from build123d import *

# Parameters (mm, degrees)
SKETCH1_W                = 30
SKETCH1_H                = 22
BOSS_EXTRUDE1_DEPTH      = 11
SKETCH2_W                = 26.5
SKETCH2_H                = 18.5
CUT_EXTRUDE1_DEPTH       = 8
SKETCH3_R                = 1.2
BOSS_EXTRUDE2_DEPTH      = 3
CUT_EXTRUDE2_DEPTH       = 2
SKETCH5_W                = 7.639048366
SKETCH5_H                = 4
CUT_EXTRUDE3_DEPTH       = 34.793490497
CUT_EXTRUDE4_REACH       = 30.81
SKETCH6_W                = 26.5
SKETCH6_H                = 2
SKETCH8_W                = 24.775890618
SKETCH8_H                = 8.79217469
CUT_EXTRUDE5_DEPTH       = 2
FILLET1_R                = 3
SKETCH10_R               = 7
SKETCH10_R_2             = 5
BOSS_EXTRUDE4_DEPTH      = 8
BOSS_EXTRUDE8_REACH      = 36.471
BOSS_EXTRUDE8_END_RADIUS = 7
SKETCH15_W               = 8
SKETCH15_H               = 10
SKETCH16_W               = 7.639048366
SKETCH16_H               = 4
CUT_EXTRUDE7_DEPTH       = 46.861094623
CUT_EXTRUDE8_REACH       = 47.861


with BuildPart() as part:
    # Sketch1 → Boss-Extrude1 (new body)
    with BuildSketch(Plane(origin=(0, 0, 0), x_dir=(1, 0, 0), z_dir=(0, 1, 0))):
        Rectangle(SKETCH1_W, SKETCH1_H)
    extrude(amount=BOSS_EXTRUDE1_DEPTH)

    # Sketch2 → Cut-Extrude1 (cut)
    with BuildSketch(Plane(origin=(0, 11, 0), x_dir=(1, 0, 0), z_dir=(0, 1, 0))):
        Rectangle(SKETCH2_W, SKETCH2_H)
    extrude(amount=-CUT_EXTRUDE1_DEPTH, mode=Mode.SUBTRACT)

    # Sketch3 → Boss-Extrude2 (add)
    with BuildSketch(Plane(origin=(0, 3, 0), x_dir=(1, 0, 0), z_dir=(0, 1, 0))):
        with Locations(Location((-10.25, -6.3, 0), (0, 0, 90))):
            Circle(SKETCH3_R)
        with Locations(Location((10.25, -6.3, 0), (0, 0, 90))):
            Circle(SKETCH3_R)
        with Locations(Location((10.25, 6.3, 0), (0, 0, 90))):
            Circle(SKETCH3_R)
        with Locations(Location((-10.25, 6.3, 0), (0, 0, 90))):
            Circle(SKETCH3_R)
    extrude(amount=BOSS_EXTRUDE2_DEPTH)

    # Sketch4 → Cut-Extrude2 (cut)
    with BuildSketch(Plane(origin=(0, 3, 0), x_dir=(1, 0, 0), z_dir=(0, 1, 0))):
        Polygon((8.552738998, 7.070702511), (8.552738998, 5.36723461), (-8.55, 5.429297489), (-8.55, 7.070702511), align=None)
    cut_extrude2 = extrude(amount=-CUT_EXTRUDE2_DEPTH, mode=Mode.SUBTRACT)

    # Mirror1: Cut-Extrude2 across plane
    add(cut_extrude2.mirror(Plane.XY), mode=Mode.SUBTRACT)

    # Sketch5 → Cut-Extrude3 (cut, through all)
    with BuildSketch(Plane.ZY.offset(15)):
        with Locations((0, 6.5)):
            Rectangle(SKETCH5_W, SKETCH5_H)
    extrude(amount=-CUT_EXTRUDE3_DEPTH, mode=Mode.SUBTRACT)

    # Sketch6 → Cut-Extrude4 (cut, up to next)
    with BuildSketch(Plane.XY.offset(11), mode=Mode.PRIVATE) as cut_extrude4_sk1:
        with Locations((0, 9)):
            Rectangle(SKETCH6_W, SKETCH6_H)
    cut_extrude4_tool1 = extrude(cut_extrude4_sk1.sketch, amount=-CUT_EXTRUDE4_REACH, mode=Mode.PRIVATE) & part.part
    add(cut_extrude4_tool1.solids().sort_by_distance((0, 9, 11))[0], mode=Mode.SUBTRACT)

    # Sketch8 → Cut-Extrude5 (cut)
    with BuildSketch(Plane(origin=(0, 3, 0), x_dir=(1, 0, 0), z_dir=(0, 1, 0))):
        Rectangle(SKETCH8_W, SKETCH8_H)
    extrude(amount=-CUT_EXTRUDE5_DEPTH, mode=Mode.SUBTRACT)

    # Fillet1
    # the kernel refuses this fillet: 3 mm, written as the material it takes off along each edge
    with BuildSketch(Plane(origin=(-15, -7.5, 11), x_dir=(1, 0, 0), z_dir=(0, 1, 0)), Plane(origin=(-15, -7.5, -11), x_dir=(0, 0, 1), z_dir=(0, 1, 0))) as fillet1_piece_1:
        with BuildLine():
            CenterArc((FILLET1_R, FILLET1_R), FILLET1_R, 180, 90)
            Line((0, FILLET1_R), (0, 0))
            Line((0, 0), (FILLET1_R, 0))
        make_face()
    extrude(amount=26, mode=Mode.SUBTRACT)
    with BuildSketch(Plane(origin=(15, -7.5, 11), x_dir=(-1, 0, 0), z_dir=(0, 1, 0)), Plane(origin=(15, -7.5, -11), x_dir=(0, 0, 1), z_dir=(0, 1, 0))) as fillet1_piece_2:
        with BuildLine():
            CenterArc((FILLET1_R, -FILLET1_R), FILLET1_R, 90, 90)
            Line((0, -FILLET1_R), (0, 0))
            Line((0, 0), (FILLET1_R, 0))
        make_face()
    extrude(amount=26, mode=Mode.SUBTRACT)



with BuildPart() as body_2:
    # Sketch10 → Boss-Extrude4 (new body)
    with BuildSketch(Plane(origin=(15, 0, -26), x_dir=(0, 0, 1), z_dir=(-1, 0, 0))):
        with Locations((26, 16.2)):
            Circle(SKETCH10_R)
        with Locations((26, 16.2)):
            Circle(SKETCH10_R_2, mode=Mode.SUBTRACT)
    extrude(amount=-BOSS_EXTRUDE4_DEPTH)


with BuildPart() as part_1:
    add(part.part)

    add(body_2.part)  # Boss-Extrude8 merges body 2
    # Boss-Extrude8: up to this cylinder (the profile starts outside it)
    boss_extrude8_end = Plane(origin=(19, 16.2, 0), z_dir=(-1, 0, 0)) * Cylinder(BOSS_EXTRUDE8_END_RADIUS, 87.942, mode=Mode.PRIVATE)
    # Sketch15 → Boss-Extrude8 (add, up to the surface)
    with BuildSketch(Plane(origin=(0, 0, 0), x_dir=(1, 0, 0), z_dir=(0, 1, 0)), mode=Mode.PRIVATE) as boss_extrude8_sk1:
        with Locations((19, 0)):
            Rectangle(SKETCH15_W, SKETCH15_H)
    boss_extrude8_tool1 = extrude(boss_extrude8_sk1.sketch, amount=BOSS_EXTRUDE8_REACH, mode=Mode.PRIVATE) - boss_extrude8_end
    add(boss_extrude8_tool1.solids().sort_by_distance((19, 0, 0))[0])

    # Sketch16 → Cut-Extrude7 (cut, through all)
    with BuildSketch(Plane(origin=(23, 0, 0), x_dir=(0, 0, -1), z_dir=(1, 0, 0))):
        with Locations((0, 6.5)):
            Rectangle(SKETCH16_W, SKETCH16_H)
    extrude(amount=-CUT_EXTRUDE7_DEPTH, mode=Mode.SUBTRACT)

    # Sketch17 → Cut-Extrude8 (cut, up to next)
    with BuildSketch(Plane(origin=(23, 0, 0), x_dir=(0, 0, -1), z_dir=(1, 0, 0)), mode=Mode.PRIVATE) as cut_extrude8_sk1:
        with BuildLine():
            Line((-4.898979486, 21.2), (-3.499271061, 19.771428571))
            ThreePointArc((-3.499271061, 19.771428571), (0.025511865, 21.199934914), (3.535533906, 19.735533906))
            Line((3.535533906, 19.735533906), (4.949747468, 21.149747468))
            ThreePointArc((4.949747468, 21.149747468), (0.03571661, 23.19990888), (-4.898979486, 21.2))
        make_face()
    cut_extrude8_tool1 = extrude(cut_extrude8_sk1.sketch, amount=-CUT_EXTRUDE8_REACH, mode=Mode.PRIVATE) & part_1.part
    add(cut_extrude8_tool1.solids().sort_by_distance((23, 21.659424, -0.027856))[0], mode=Mode.SUBTRACT)


solid = part_1.part
Build history of the part. All positions in model axes, mm. A direction names the side the tool comes from. Coordinates: 2 decimals unless noted, no trailing zeros. Order: outer loops, then holes, each group sorted by start corner. A loop starts at its lowest first (then second) coordinate and runs counter-clockwise, first axis right, second up. Notation, with made-up numbers: M 55,39 L 93,39 A24 cw 93,70 Z; hole C 38,-11.75 d5. An arc over 180 degrees is marked long. One line per question, with ' | ' between items. Start each with the question number.
Q1. Saw through at A-A (y = 1.5). List the corners of the cut face in (x, z), then the cut area to 3 significant figures.
Q2. Two-plate mould, pull along Z, no slides. Class faces 5 (the face through (23, 10, 0)), 6 (the face through (18.9, 16.2, 7)), 7 (the face through (-14, 6, 3.82)): +Z half, -Z half, draft (parallel to the pull), parting line (faces both ways), or undercut.
Q3. Saw through at B-B (z = 0). List the corners of the cut face in (x, y), then the cut area to 3 significant figures.
Q4. Saw through at C-C (x = -10.25). List the corners of the cut face in (y, z), then the cut area to 3 significant figures.
Q5. Flat gauge pins, fed straight in: pin 1 Ø2.5 at (x, z) = (10.5, -6.5) entering from +Y; pin 2 Ø3 at (x, y) = (0, 11.5) entering from -Z; pin 3 Ø1.9 at (x, z) = (0, 6.5) entering from +Y; pin 4 Ø1.5 at (x, y) = (15.5, 11) entering from -Z. Where does each tip first touch, or does it go through?
Q6. Probe L1, parallel to X at y = 9, z = -4.25; L2, parallel to Z at x = -10.5, y = 2; L3, parallel to Y at x = 18.25, z = 0. List the from-to ranges inside material, lowest first. Write a range as from..to.
Q7. Saw through at D-D (y = 16.2). List the corners of the cut face in (x, z), then the cut area to 3 significant figures.
Q8. 3-axis set-ups, long thin cutter, end or side, ignore diameter. For faces 1 (the face through (0, 8, 10)), 2 (the face through (19, 6, -5)), 3 (the face through (0, 11, 10)), 4 (the face through (0, 1, 0)): which of +Z, -Z, +X, -X, +Y, -Y reach the whole face in a straight line?
Check values:
1) outline: M -15,-8 A3 ccw -12,-11 L 12,-11 A3 ccw 15,-8 L 15,-5 L 23,-5 L 23,5 L 15,5 L 15,8 A3 ccw 12,11 L -12,11 A3 ccw -15,8 Z; hole M -12.39,-4.4 L 12.39,-4.4 L 12.39,4.4 L -12.39,4.4 Z; hole M -8.55,-7.07 L 8.55,-7.07 L 8.55,-5.37 L -8.55,-5.43 Z; hole M -8.55,5.43 L 8.55,5.37 L 8.55,7.07 L -8.55,7.07 Z | area: 457 mm2
2) face 5: draft | face 6: +Z half | face 7: undercut
3) outline: M -15,0 L 23,0 L 23,4.5 L 13.25,4.5 L 13.25,3 L 12.39,3 L 12.39,1 L -12.39,1 L -12.39,3 L -13.25,3 L -13.25,4.5 L -15,4.5 Z; M -15,8.5 L -13.25,8.5 L -13.25,11 L -15,11 Z; M 13.25,8.5 L 23,8.5 L 23,11.2 L 15,11.2 L 15,11 L 13.25,11 Z | area: 112 mm2
4) outline: M 0,-11 L 11,-11 L 11,-9.25 L 3,-9.25 L 3,-7.5 L 6,-7.5 L 6,-5.1 L 3,-5.1 L 3,-4.4 L 1,-4.4 L 1,4.4 L 3,4.4 L 3,5.1 L 6,5.1 L 6,7.5 L 3,7.5 L 3,9.25 L 8,9.25 L 8,11 L 0,11 Z; M 10,9.25 L 11,9.25 L 11,11 L 10,11 Z | area: 87.3 mm2
5) pin 1: stops at y = 6 | pin 2: stops at z = -11 | pin 3: stops at y = 3 | pin 4: stops at z = -9.2
6) L1: x = -15..-13.25, 13.25..23 | L2: z = -11..-4.4, 4.4..11 | L3: y = 0..4.5, 8.5..11.2
7) outline: M 15,-7 L 23,-7 L 23,-5 L 15,-5 Z; M 15,5 L 23,5 L 23,7 L 15,7 Z | area: 32.0 mm2
8) face 1: +Z | face 2: -Z, +X, -Y | face 3: +Z, -Z, -X, +Y | face 4: +Y
